Could you check a few things on this model? Use its own coordinates, in mm. A direction names the side the tool comes from. Coordinates: 2 decimals unless noted, no trailing zeros. Order: outer loops, then holes, each group sorted by start corner. A loop starts at its lowest first (then second) coordinate and runs counter-clockwise, first axis right, second up.
```python
from build123d import *

# Parameters (mm, degrees)
F0_R     = 38.1
F0_R_2   = 31.75
F1_DEPTH = 123.825
F2_DEPTH = 114.3


# Not quite as in the source:
# - a fillet or chamfer that OpenCascade refuses, or shapes differently, is made with other operations: its cross-section is extruded or revolved along the edge and cut away or added


with BuildPart() as f1:
    # F0 (on Top) → F1 (new body)
    with BuildSketch(Plane.XY):
        Circle(F0_R)
        Circle(F0_R_2, mode=Mode.SUBTRACT)
        Circle(F0_R_2)
    extrude(amount=-F1_DEPTH)

    # F0 (on Top) → F2 (cut)
    with BuildSketch(Plane.XY):
        Circle(F0_R_2)
    extrude(amount=-F2_DEPTH, mode=Mode.SUBTRACT)

    # F3: fillet of radius 12.7 on 1 edges, made by hand

    # F3_s1 → F3_t2 (revolve, cut)
    with BuildSketch(Plane.XZ):
        with BuildLine():
            ThreePointArc((38.1, -10.9985226281), (36.3985226281, -4.6485226281), (31.75, 0))
            Line((31.75, 0), (38.1, 0))
            Line((38.1, 0), (38.1, -10.9985226281))
        make_face()
    revolve(axis=Axis((0, 0, 0), (0, 0, 1)), mode=Mode.SUBTRACT)


solid = f1.part
```
Item 1: Suppose I cut it at C-C (z = -103.5). List the corners of the cut face in (x, y) for me, and give its area (3 significant figures).
Item 2: Which directions (+Z, -Z, +X, -X, +Y, -Y) give clear straight access to the entire face, cutting with the end or side of a thin tool? Please do faces 1 (the face through (-30.235, -23.183, -66.622)), 2 (the face through (-6.883, -30.995, -56.35)).
Item 3: For pin 1 Ø3 at (x, z) = (24, -18.5) entering from +Y; pin 2 Ø19 at (x, y) = (-10, 9) entering from +Z; pin 3 Ø5 at (x, z) = (24.5, -26.5) entering from -Y, each with a flat end and sliding along its axis, tell me the tip position at first contact or that it passes through.
Item 4: I need wall thicknesses on line 1 (Y direction, x = 0, z = -57); line 2 (Z direction, x = -13, y = -20) (3 decimals); line 3 (Y direction, x = -23, z = -109.5). Which ranges of each line are inside material? Lowest first, please.
Item 5: Suppose I cut it at A-A (x = 0). List the corners of the cut face in (y, z) for me (3 decimals), and give its area (3 significant figures).
Geometry results:
1. outline: circle Ø76.2 at (0, 0); hole circle Ø63.5 at (0, 0)
1. area: 1,390 mm2
2. face 1: +Z, -Z
2. face 2: +Z
3. pin 1: stops at y = 30.75
3. pin 2: stops at z = -114.3
3. pin 3: stops at y = -31.11
4. line 1: y = -38.1 to -31.75, 31.75 to 38.1
4. line 2: z = -123.825 to -114.3
4. line 3: y = -30.37 to -21.89, 21.89 to 30.37
5. outline: (-38.1, -123.825) - (38.1, -123.825) - (38.1, -10.999) arc R12.7 ccw to (31.75, 0) - (31.75, -114.3) - (-31.75, -114.3) - (-31.75, 0) arc R12.7 ccw to (-38.1, -10.999) - close
5. area: 2,140 mm2
